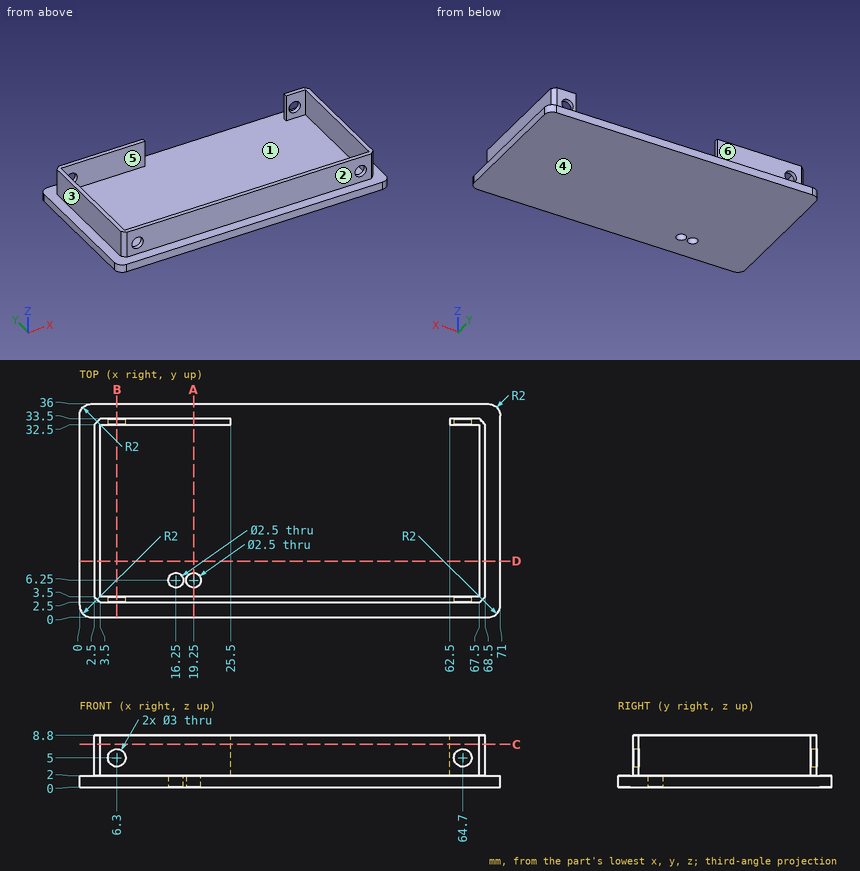
Geometry: see drawing. Coordinates: mm, zero at the bounding-box minimum. A direction names the side the tool comes from. Round coordinates to 2 decimals unless told otherwise and drop trailing zeros. Write each loop counter-clockwise with the first axis right and the second up, starting at its lowest first coordinate (ties: lowest second). Pieces come first, ordered by that corner, then holes.
Item 1: Mould query, pull axis Y, two halves, no side actions, for the marked faces 4, 5 and 6. Classes: +Y half, -Y half, draft (parallel to the pull), parting line (faces both ways), or undercut.
Item 2: Section query A-A (x = 19.25). Return loops of the section in (y, z).
Item 3: Section query B-B (x = 6.3). Return loops of the section in (y, z), plus the area to 3 significant figures.
Item 4: Pin query (flat end, axial travel): P1, Ø2.5, axis at x = 64.7, z = 5, coming from the -Y side; P2, Ø2, axis at x = 25, y = 24.5, coming from the +Z side; P3, Ø3.5, axis at y = 24, z = 4, coming from the +X side; P4, Ø3.5, axis at x = 35, z = 5.5, coming from the +Y side. Return the tip coordinate at first contact, or that it passes through.
Item 5: Material intervals for L1, parallel to X at y = 19, z = 4.25; L2, parallel to Z at x = 6.3, y = 3; L3, parallel to X at y = 6.25, z = 0.55, sorted ascending.
Item 6: Section query C-C (z = 7.25). Return loops of the section in (x, y).
Item 7: Set-up query: the marked faces 1, 2 and 3. Return all of +Z, -Z, +X, -X, +Y, -Y with unobstructed straight access to the full face (end or side cutting, diameter ignored); none if empty.
Item 8: Section query D-D (y = 9.5). Return loops of the section in (x, z).
Completed:
1. face 4: draft
1. face 5: undercut
1. face 6: +Y half
2. outline: (0, 0) - (5, 0) - (5, 2) - (3.5, 2) - (3.5, 8.8) - (2.5, 8.8) - (2.5, 2) - (0, 2) - close; (7.5, 0) - (36, 0) - (36, 2) - (33.5, 2) - (33.5, 8.8) - (32.5, 8.8) - (32.5, 2) - (7.5, 2) - close
3. outline: (0, 0) - (36, 0) - (36, 2) - (33.5, 2) - (33.5, 3.5) - (32.5, 3.5) - (32.5, 2) - (3.5, 2) - (3.5, 3.5) - (2.5, 3.5) - (2.5, 2) - (0, 2) - close; (2.5, 6.5) - (3.5, 6.5) - (3.5, 8.8) - (2.5, 8.8) - close; (32.5, 6.5) - (33.5, 6.5) - (33.5, 8.8) - (32.5, 8.8) - close
3. area: 79.6 mm2
4. P1: passes through
4. P2: stops at z = 2
4. P3: stops at x = 68.5
4. P4: stops at y = 3.5
5. L1: x = 2.5 to 3.5, 67.5 to 68.5
5. L2: z = 0 to 3.5, 6.5 to 8.8
5. L3: x = 0 to 15, 17.5 to 18, 20.5 to 71
6. outline: (2.5, 3.5) - (3.5, 2.5) - (67.5, 2.5) - (68.5, 3.5) - (68.5, 32.5) - (67.5, 33.5) - (62.5, 33.5) - (62.5, 32.5) - (67.5, 32.5) - (67.5, 3.5) - (3.5, 3.5) - (3.5, 32.5) - (25.5, 32.5) - (25.5, 33.5) - (3.5, 33.5) - (2.5, 32.5) - close
7. face 1: +Z
7. face 2: +Z, +X, -X, -Y
7. face 3: +Z, -X, +Y, -Y
8. outline: (0, 0) - (71, 0) - (71, 2) - (68.5, 2) - (68.5, 8.8) - (67.5, 8.8) - (67.5, 2) - (3.5, 2) - (3.5, 8.8) - (2.5, 8.8) - (2.5, 2) - (0, 2) - close
